Check sheet for the drawn part. Datum: minimum x, y, z corner. Units: mm. A direction names the side the tool comes from. Round coordinates to 2 decimals unless told otherwise and drop trailing zeros. Write each loop counter-clockwise with the first axis right and the second up, starting at its lowest first coordinate (ties: lowest second). Pieces come first, ordered by that corner, then holes. Notation, with made-up numbers: (-26.75, 88) - (-0.75, 88) arc R8 ccw to (-0.75, 92) - close; hole circle Ø5 at (-1, -2.75). An arc over 180 degrees is marked (long way). Answer as a JSON object with one key per item and string values.
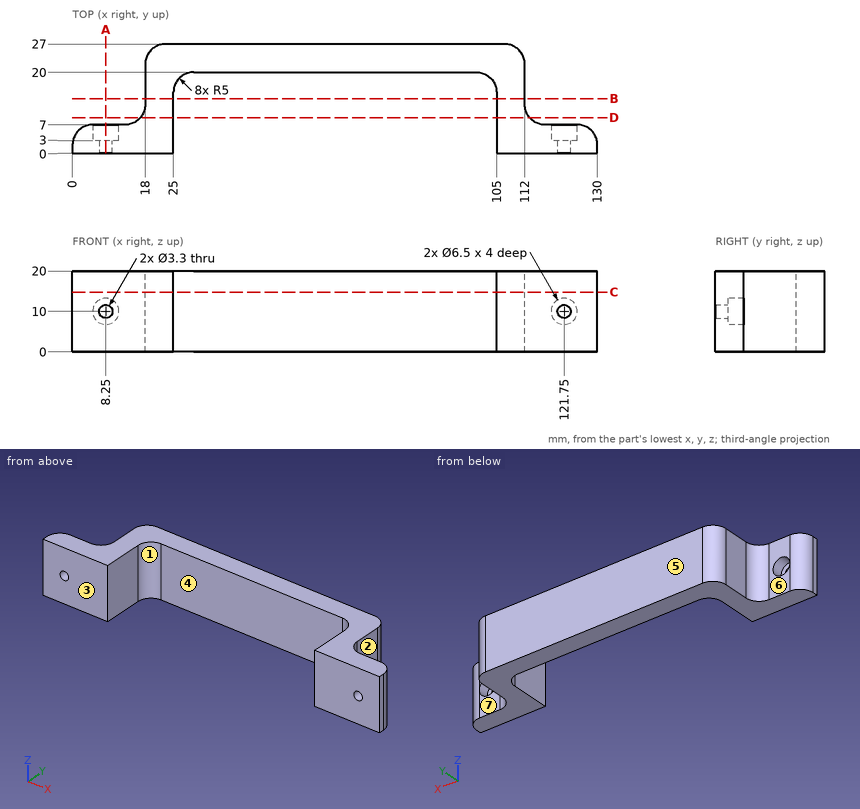
1. Cross-section at C-C (z = 14.75). Record the boundary of the cut face in (x, y).
Completed:
{"outline": "(0, 0) - (25, 0) - (25, 15) arc R5 cw to (30, 20) - (100, 20) arc R5 cw to (105, 15) - (105, 0) - (130, 0) - (130, 2) arc R5 ccw to (125, 7) - (117, 7) arc R5 cw to (112, 12) - (112, 22) arc R5 ccw to (107, 27) - (23, 27) arc R5 ccw to (18, 22) - (18, 12) arc R5 cw to (13, 7) - (5, 7) arc R5 ccw to (0, 2) - close"}
2. Mould release check, pull along X, two halves, no side actions. Record for the marked faces 1, 2 and 3: released by +X, released by -X, zero draft, split by the parting line, or undercut.
Completed:
{"face 1": "undercut", "face 2": "released by +X", "face 3": "zero draft"}
3. Cross-section at A-A (x = 8.25). Record the boundary of the cut face in (y, z).
Completed:
{"outline": "(0, 0) - (7, 0) - (7, 6.75) - (3, 6.75) - (3, 8.35) - (0, 8.35) - close; (0, 11.65) - (3, 11.65) - (3, 13.25) - (7, 13.25) - (7, 20) - (0, 20) - close"}
4. Access from +Z, -Z, +X, -X, +Y, -Y to the whole of each face (thin tool, end or side, straight path). Record for the marked faces 4, 5, 6 and 7.
Completed:
{"face 4": "+Z, -Z, -Y", "face 5": "+Z, -Z, +X, -X, +Y", "face 6": "+Z, -Z, -X, +Y", "face 7": "+Z, -Z, +X, +Y"}
5. Cross-section at B-B (y = 13.5). Record the boundary of the cut face in (x, z).
Completed:
{"outline": "(18, 0) - (25, 0) - (25, 20) - (18, 20) - close; (105, 0) - (112, 0) - (112, 20) - (105, 20) - close"}
6. Material ranges on probe 1 along Z at (x, y) = (121.75, 5); probe 2 along Z at (x, y) = (121.75, 2.4); probe 3 along X at (y, z) = (1, 6.5), recorded low to high. Write a range as from..to.
Completed:
{"probe 1": "z = 0..6.75, 13.25..20", "probe 2": "z = 0..8.35, 11.65..20", "probe 3": "x = 0..25, 105..130"}
7. Go/stop test with flat-tipped pins: pin 1 (7.5 mm diameter, centred on x = 8.25, z = 10, fed in from +Y); pin 2 (5 mm diameter, centred on y = 5, z = 14.5, fed in from +X); pin 3 (4 mm diameter, centred on x = 121.75, z = 10, fed in from +Y); pin 4 (10 mm diameter, centred on x = 16.5, y = 6.5, fed in from -Z). Record where each tip stops, or that it passes through.
Completed:
{"pin 1": "stops at y = 7", "pin 2": "stops at x = 129.97", "pin 3": "stops at y = 3", "pin 4": "stops at z = 0"}
8. Cross-section at D-D (y = 8.75). Record the boundary of the cut face in (x, z), plus the area to 3 significant figures.
Completed:
{"outline": "(16.8, 0) - (25, 0) - (25, 20) - (16.8, 20) - close; (105, 0) - (113.2, 0) - (113.2, 20) - (105, 20) - close", "area": "328 mm^2"}
